Verification items for the finished model (mm, model axes). Face numbers are marked on the shaded views. A direction names the side the tool comes from. Coordinates: 2 decimals unless noted, no trailing zeros. Order: outer loops, then holes, each group sorted by start corner. A loop starts at its lowest first (then second) coordinate and runs counter-clockwise, first axis right, second up. Notation, with made-up numbers: (24, 36.5) -> (83, 36.5) arc R23 ccw to (83, 62.5) -> close; hole circle Ø9 at (41.5, 63.25). An arc over 180 degrees is marked (long way). Write item = value, one per line. Start each with the question number.
Autodesk Inventor part; units mm, degrees
ref_plane "YZ Plane" through (0, 0, 0) normal (1, 0, 0) x (0, 1, 0)
ref_plane "XZ Plane" through (0, 0, 0) normal (0, 1, 0) x (-1, 0, 0)
ref_plane "XY Plane" through (0, 0, 0) normal (0, 0, 1) x (1, 0, 0)
sketch "Sketch1" plane through (0, 0, 0) normal (0, 1, 0) x (-1, 0, 0)
  line L0 (9.4, 9.575) -> (-9.4, 9.575)
  line L1 (-9.4, 9.575) -> (-9.4, -9.575)
  line L2 (-9.4, -9.575) -> (9.4, -9.575)
  line L3 (9.4, -9.575) -> (9.4, 9.575)
  line L4 (9.4, 9.575) -> (-9.4, -9.575) construction
  line L5 (-9.4, 9.575) -> (9.4, -9.575) construction
  point P0 (0, 0)
  dimension "d0" = 18.8
  dimension "d1" = 19.15
extrude "Extrusion1" add sketch "Sketch1" along normal blind 11.61
sketch "Sketch6" plane through (9.4, 0, 9.575) normal (1, 0, 0) x (0, 0, -1)
  line L0 (0, 0) -> (19.15, 0)
  line L1 (0, 0) -> (0, 11.61)
  line L2 (19.15, 0) -> (19.15, 11.61)
  point P0 (9.575, 0)
  point P1 (14.15, 5.44)
  dimension "d60" = 5.44
  dimension "d76" = 5
hole "Hole6" at (9.4, 5.44, -4.575) direction (-1, 0, 0) diameter 4.077 depth 5
sketch "Sketch7" plane through (-9.4, 0, -9.575) normal (-1, 0, 0) x (0, 0, 1)
  circle A0 centre (5, 5.44) radius 2.0385
  point P0 (9.575, 0)
hole "Hole7" at (-9.4, 5.44, -4.575) direction (1, 0, 0) diameter 4.077 depth 5
sketch "Sketch8" plane through (0, 11.61, 0) normal (0, 1, 0) x (1, 0, 0)
  line L0 (-37.5313, 24.2217) -> (38.0409, 24.2217) construction
  line L1 (38.0409, 24.2217) -> (38.0409, -24.8493) construction
  line L2 (38.0409, -24.8493) -> (-37.5313, -24.8493) construction
  line L3 (-37.5313, -24.8493) -> (-37.5313, 24.2217) construction
  point P0 (0, 0)
sketch "Sketch9" plane through (0, 0, 0) normal (0, -1, 0) x (1, 0, 0)
  line L0 (2.285, 15.035) -> (-2.285, 15.035)
  line L1 (-2.285, 15.035) -> (-2.285, -15.035)
  line L2 (-2.285, -15.035) -> (2.285, -15.035)
  line L3 (2.285, -15.035) -> (2.285, 15.035)
  line L4 (2.285, 15.035) -> (-2.285, -15.035) construction
  line L5 (-2.285, 15.035) -> (2.285, -15.035) construction
  point P0 (0, 0)
  dimension "d77" = 4.57
  dimension "d78" = 30.07
extrude "Extrusion2" add sketch "Sketch9" against normal blind 1.02
sketch "Sketch10" plane through (0, 0, 0) normal (0, -1, 0) x (1, 0, 0)
  line L0 (-2.285, -15.035) -> (2.285, -15.035) construction
  line L1 (0, -15.035) -> (0, 15.035) construction
  line L2 (-2.285, 15.035) -> (2.285, 15.035) construction
  point P0 (0, 0)
  point P1 (0, -12.7)
  point P2 (0, 12.7)
  dimension "d81" = 12.7
  dimension "d82" = 12.7
hole "Hole8" at (0, 0, -12.7) at (0, 0, 12.7) direction (0, 1, 0) diameter 2.7 end through all
sketch "Sketch11" plane through (-9.4, 0, -9.575) normal (-1, 0, 0) x (0, 0, 1)
  circle A0 centre (11.4, 8.31) radius 1
  circle A1 centre (14.86, 5.44) radius 1
  line L0 (0, 0) -> (19.15, 0)
  line L1 (0, 0) -> (0, 11.61)
  point P0 (9.575, 0)
  dimension "d90" = 2
  dimension "d91" = 2
  dimension "d92" = 5.44
  dimension "d93" = 8.31
  dimension "d94" = 14.86
  dimension "d95" = 11.4
extrude "Extrusion3" add sketch "Sketch11" along normal blind 4
sketch "Sketch12" plane through (0, 11.61, 0) normal (0, 1, 0) x (1, 0, 0)
  line L0 (-9.3536, 9.4666) -> (9.2116, 9.4666) construction
  line L1 (9.2116, 9.4666) -> (9.2116, -9.4331) construction
  line L2 (9.2116, -9.4331) -> (-9.3536, -9.4331) construction
  line L3 (-9.3536, -9.4331) -> (-9.3536, 9.4666) construction
properties part number "USB-1SP16T-83H-01"
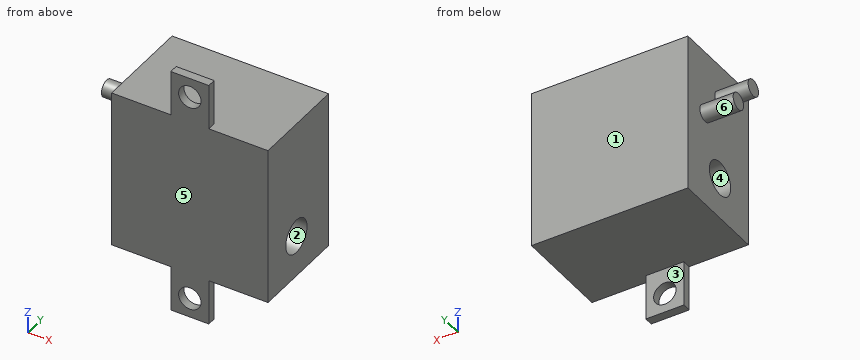
Item 1: Gauge pin test, flat ends, axial feed: P1, Ø1.4, axis at x = 0.5, z = -12, coming from the +Y side; P2, Ø4.5, axis at y = 5, z = -4.5, coming from the +X side; P3, Ø6, axis at x = -10.5, y = 6, coming from the +Z side (3 decimals); P4, Ø4, axis at x = -6.5, y = 1.5, coming from the -Z side (3 decimals). Record the tip position at first contact, or that the pin passes through.
Item 2: Section check C-C (y = 8.31). Record the boundary of the cut face in (x, z) (3 decimals).
Item 3: Tool access check on the marked faces 1 and 2. Record the directions out of +Z, -Z, +X, -X, +Y, -Y that give a thin tool (end or side, any length) a straight path to the whole face; none if there is none.
Item 4: Section check B-B (z = -12.7). Record the boundary of the cut face in (x, y) (3 decimals).
Item 5: Thickness scan on line 1 (X direction, y = 0.3, z = -12.7) (3 decimals); line 2 (Z direction, x = 8.3, y = 5.44) (1 decimal); line 3 (Z direction, x = 0, y = 0.55) (3 decimals). Record the ranges inside material, lowest first.
Item 6: Mould release check, pull along Y, two halves, no side actions. Record for the marked faces 3, 4, 5 and 6: pulls with the +Y half, pulls with the -Y half, needs draft (parallel to the pull), parting line crosses it, or undercut.
Item 7: Section check A-A (x = 0). Record the boundary of the cut face in (y, z) (3 decimals), then the cut area to 3 significant figures.
Item 8: Section check D-D (z = -1.5). Record the boundary of the cut face in (x, y).
Filled sheet:
q1.P1 = 1.02
q1.P2 = 9.4
q1.P3 = 9.575
q1.P4 = -9.575
q2.outline = (-13.4, 0.825) -> (-9.4, 0.825) -> (-9.4, -9.575) -> (9.4, -9.575) -> (9.4, 9.575) -> (-9.4, 9.575) -> (-9.4, 2.825) -> (-13.4, 2.825) -> close
q3.face_1 = +Z, -Z, +X, -X, +Y
q3.face_2 = +X
q4.outline = (-2.285, 0) -> (-1.35, 0) -> (-1.35, 1.02) -> (-2.285, 1.02) -> close; (1.35, 0) -> (2.285, 0) -> (2.285, 1.02) -> (1.35, 1.02) -> close
q5.line_1 = -2.285 to -1.35, 1.35 to 2.285
q5.line_2 = -9.6 to -6.6, -2.5 to 9.6
q5.line_3 = -15.035 to -14.05, -11.35 to 11.35, 14.05 to 15.035
q6.face_3 = pulls with the +Y half
q6.face_4 = undercut
q6.face_5 = pulls with the -Y half
q6.face_6 = parting line crosses it
q7.outline = (0, -15.035) -> (1.02, -15.035) -> (1.02, -14.05) -> (0, -14.05) -> close; (0, -11.35) -> (1.02, -11.35) -> (1.02, -9.575) -> (11.61, -9.575) -> (11.61, 9.575) -> (1.02, 9.575) -> (1.02, 11.35) -> (0, 11.35) -> close; (0, 14.05) -> (1.02, 14.05) -> (1.02, 15.035) -> (0, 15.035) -> close
q7.area = 228 mm^2
q8.outline = (-9.4, 0) -> (9.4, 0) -> (9.4, 11.61) -> (-9.4, 11.61) -> close
